Verification items for this drawing (mm, ordinates from the low corner). A direction names the side the tool comes from. Round coordinates to 2 decimals unless told otherwise and drop trailing zeros. Loops run counter-clockwise (first coordinate to the right, second up) from the corner with the lowest first, then second, coordinate; pieces in that order, holes last. Notation, with made-up numbers: M -25.75,53 L 26.25,53 A36 ccw 26.25,91 Z; hole C 9,57 d6. An arc over 180 degrees is marked long. Answer as CSV lines item,"result".
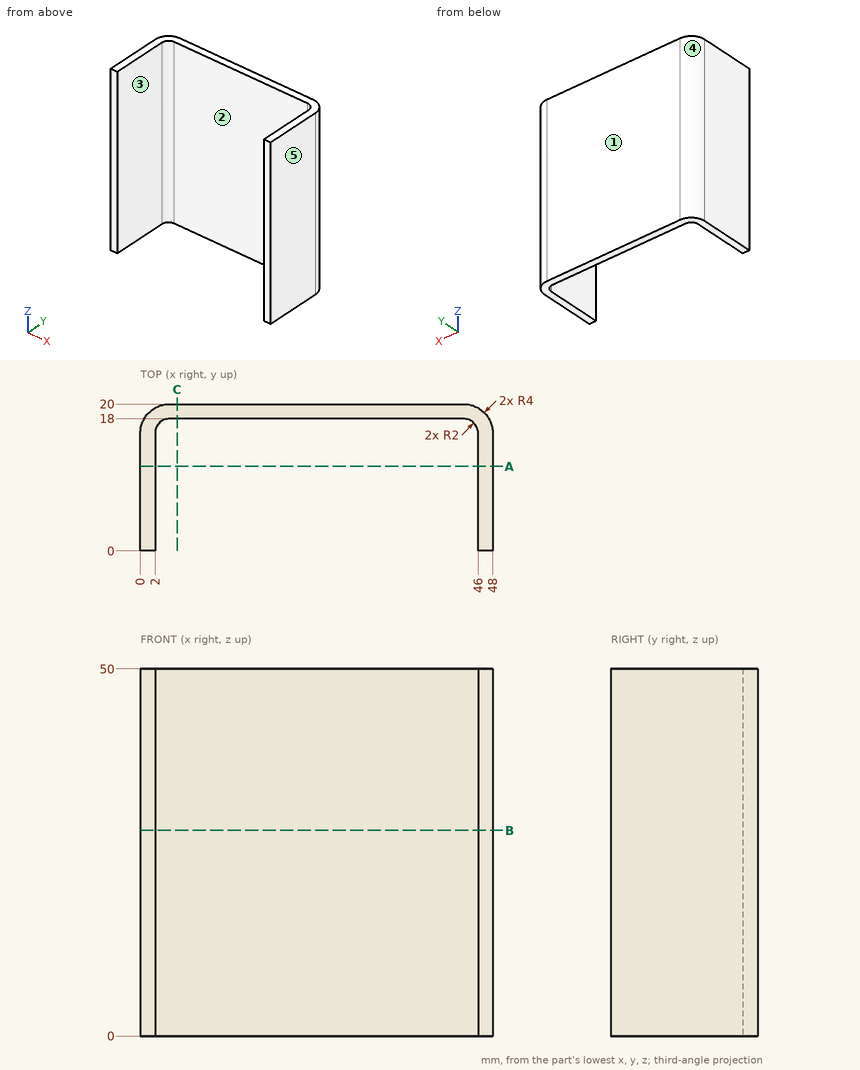
1) Go/stop test with flat-tipped pins: pin 1 (5 mm diameter, centred on x = 43, z = 8.5, fed in from -Y); pin 2 (10 mm diameter, centred on x = 29.5, z = 7, fed in from -Y). Record where each tip stops, or that it passes through.
Here are the results:
pin 1,"stops at y = 17.32"
pin 2,"stops at y = 18"
2) Section check A-A (y = 11.5). Record the cut outline in (x, z).
Here are the results:
outline,"M 0,0 L 2,0 L 2,50 L 0,50 Z; M 46,0 L 48,0 L 48,50 L 46,50 Z"
3) Set-up check for the marked faces 1 and 2: record each of +Z, -Z, +X, -X, +Y, -Y from which the full face is reachable in a straight line by a thin tool's end or side.
Here are the results:
face 1,"+Z, -Z, +X, -X, +Y"
face 2,"+Z, -Z, -Y"
4) Material ranges on probe 1 along X at (y, z) = (14.5, 20); probe 2 along Y at (x, z) = (12, 32.5); probe 3 along X at (y, z) = (16.5, 34.5), recorded low to high.
Here are the results:
probe 1,"x = 0 to 2, 46 to 48"
probe 2,"y = 18 to 20"
probe 3,"x = 0.03 to 2.06, 45.94 to 47.97"
5) Section check B-B (z = 28). Record the cut outline in (x, y), plus the area to 3 significant figures.
Here are the results:
outline,"M 0,0 L 2,0 L 2,16 A2 cw 4,18 L 44,18 A2 cw 46,16 L 46,0 L 48,0 L 48,16 A4 ccw 44,20 L 4,20 A4 ccw 0,16 Z"
area,"163 mm^2"
6) Draft check along X on the marked faces 3, 4 and 5. Enter one of: +X half, -X half, draft (parallel to the pull), parting line (faces both ways), or undercut.
Here are the results:
face 3,"undercut"
face 4,"-X half"
face 5,"+X half"
7) Section check C-C (x = 5). Record the cut outline in (y, z), plus the area to 3 significant figures.
Here are the results:
outline,"M 18,0 L 20,0 L 20,50 L 18,50 Z"
area,"100 mm^2"
